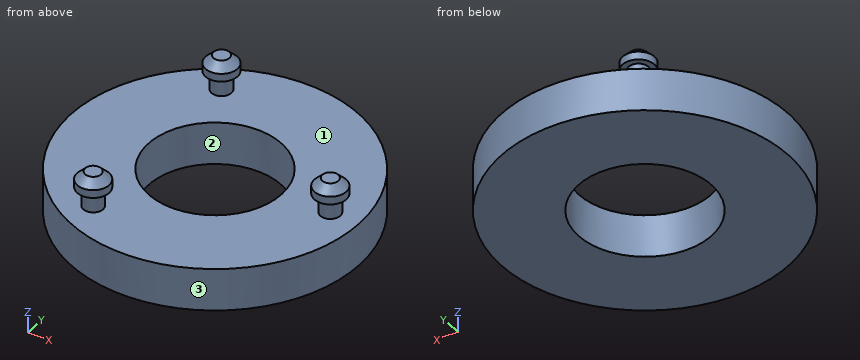
```python
from build123d import *

# Parameters (mm, degrees)
SKETCH012_R     = 27
SKETCH012_R_2   = 12.5
PAD003_DEPTH    = 8
SKETCH013_R     = 1.875
PAD004_DEPTH    = 3.6
SKETCH014_R     = 3
PAD005_DEPTH    = 3
CHAMFER004_SIZE = 1.5


with BuildPart() as part:
    # Sketch012 → Pad003 (new body)
    with BuildSketch(Plane.XY):
        Circle(SKETCH012_R)
        Circle(SKETCH012_R_2, mode=Mode.SUBTRACT)
    extrude(amount=-PAD003_DEPTH)

    # Sketch013 → Pad004 (join)
    with BuildSketch(Plane.XY):
        with Locations((-10.75, 18.619546)):
            Circle(SKETCH013_R)
        with Locations((-10.75, -18.619546)):
            Circle(SKETCH013_R)
        with Locations((21.5, 0)):
            Circle(SKETCH013_R)
    extrude(amount=PAD004_DEPTH)

    # Sketch014 (on DatumPlane) → Pad005 (join)
    with BuildSketch(Plane.XY.offset(3.6)):
        with Locations((-10.75, 18.619546)):
            Circle(SKETCH014_R)
        with Locations((21.5, 0)):
            Circle(SKETCH014_R)
        with Locations((-10.75, -18.619546)):
            Circle(SKETCH014_R)
    extrude(amount=PAD005_DEPTH)

    # Chamfer004
    chamfer004_edges = [part.edges().sort_by_distance(p)[0] for p in [
        (18.5, 0, 6.6),
        (-13.75, 18.619546, 6.6),
        (-13.75, -18.619546, 6.6),
    ]]
    chamfer(chamfer004_edges, length=CHAMFER004_SIZE)


with BuildPart() as part_1:
    # Body001 placement: moved
    add(part.part.moved(Location((0, 11, -28))))


solid = part_1.part
```
Source: CAD feature listing. Evaluate the final solid. Frame: model axes, mm. Face numbers are marked on the shaded views. Give positions to 0.01 mm unless a question says otherwise; leave off trailing zeros. Write each loop counter-clockwise with the first axis right and the second up, starting at its lowest first coordinate (ties: lowest second). Pieces come first, ordered by that corner, then holes.
1. Pull-direction query (X, two-part tool) for the marked faces 1, 2 and 3; classes: +X half, -X half, draft (parallel to the pull), parting line (faces both ways), or undercut.
2. Material intervals for line 1 along Y through (x, z) = (0, -32.5); line 2 along Z through (x, y) = (-15.5, 15); line 3 along X through (y, z) = (5, -31.5), sorted ascending.
3. Section query D-D (z = -30.5). Return the cut outline in (x, y).
4. Section query A-A (y = 16.5). Return the cut outline in (x, z).
5. Section query C-C (y = 11). Return the cut outline in (x, z) (3 decimals).
6. Section query B-B (x = 0). Return the cut outline in (y, z).
7. First-contact query: pin 1 (20 mm diameter, centred on x = 0, y = 11, fed in from -Z); pin 2 (6 mm diameter, centred on x = 9.5, z = -34.5, fed in from -Y); pin 3 (8 mm diameter, centred on y = -5.5, z = -28, fed in from -X); pin 4 (2 mm diameter, centred on x = 4.5, z = -30, fed in from +Y). Flat tips, straight axial feed; report the tip coordinate or a pass-through.
Output values:
1. face 1: draft
1. face 2: undercut
1. face 3: parting line
2. line 1: y = -16 to -1.5, 23.5 to 38
2. line 2: z = -36 to -28
2. line 3: x = -26.32 to -10.97, 10.97 to 26.32
3. outline: circle Ø54 at (0, 11); hole circle Ø25 at (0, 11)
4. outline: (-26.43, -36) - (-11.22, -36) - (-11.22, -28) - (-26.43, -28) - close; (11.22, -36) - (26.43, -36) - (26.43, -28) - (11.22, -28) - close
5. outline: (-27, -36) - (-12.5, -36) - (-12.5, -28) - (-27, -28) - close; (12.5, -36) - (27, -36) - (27, -28) - (23.375, -28) - (23.375, -24.4) - (24.5, -24.4) - (24.5, -22.9) - (23, -21.4) - (20, -21.4) - (18.5, -22.9) - (18.5, -24.4) - (19.625, -24.4) - (19.625, -28) - (12.5, -28) - close
6. outline: (-16, -36) - (-1.5, -36) - (-1.5, -28) - (-16, -28) - close; (23.5, -36) - (38, -36) - (38, -28) - (23.5, -28) - close
7. pin 1: passes through
7. pin 2: stops at y = -15.21
7. pin 3: stops at x = -23.93
7. pin 4: stops at y = 37.77
